Job drawing, mm, ordinate dimensions from the low corner. One solid piece. A direction names the side the tool comes from. Round coordinates to 2 decimals unless told otherwise and drop trailing zeros. Return JSON: item names as keys, results as strings. Group by question number.
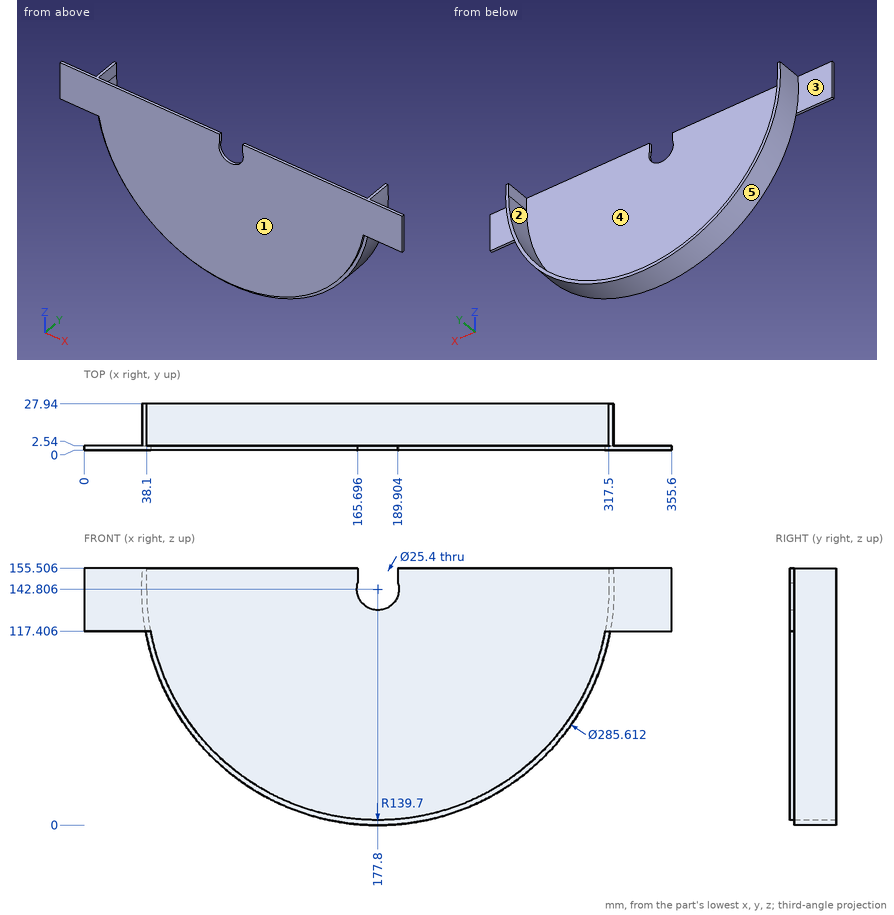
(1) Tool access for the marked faces 1 and 2: list every direction of +Z, -Z, +X, -X, +Y, -Y with a clear straight run to the whole face (end or side of a thin tool).
(2) Mould opens along X. For the marked faces 3, 4 and 5 say: pulls with the +X half, pulls with the -X half, needs draft (parallel to the pull), parting line crosses it, or undercut.
(3) Pin check, flat tips, straight feed: P1, Ø4, axis at y = 23, z = 68, coming from the +X side; P2, Ø6.5, axis at y = 11.5, z = 149, coming from the +X side (1 decimal); P3, Ø2, axis at y = 11.5, z = 118.5, coming from the +X side. Stop position of each tip, or through.
(4) Probe L1, parallel to Y at x = 133, z = 140; L2, parallel to Z at x = 177.8, y = 1.4 (1 decimal); L3, parallel to X at y = 15.25, z = 59. List the from-to ranges inside material, lowest first. Write a range as [from, to].
Results are:
{
 "1": {"face 1": "+Z, -Z, +X, -X, -Y", "face 2": "+Z, +Y"},
 "2": {"face 3": "needs draft", "face 4": "undercut", "face 5": "parting line crosses it"},
 "3": {"P1": "stops at x = 300.65", "P2": "stops at x = 320.6", "P3": "stops at x = 318.69"},
 "4": {"L1": "y = [0, 2.54]", "L2": "z = [3.1, 130.1]", "L3": "x = [62.17, 66.03], [289.57, 293.43]"}
}
